Part model, mm, in its own coordinate system. A direction names the side the tool comes from. Give positions to 0.01 mm unless a question says otherwise; leave off trailing zeros. Order: outer loops, then holes, each group sorted by start corner. A loop starts at its lowest first (then second) coordinate and runs counter-clockwise, first axis right, second up. Notation, with made-up numbers: M 16.25,-2 L 38.25,-2 A9 ccw 38.25,12 Z; hole C 37.5,-9 d1. An arc over 180 degrees is marked long. One line per question, with ' | ' between items.
Autodesk Inventor part; units mm, degrees
ref_plane "YZ Plane" through (0, 0, 0) normal (1, 0, 0) x (0, 1, 0)
ref_plane "XZ Plane" through (0, 0, 0) normal (0, 1, 0) x (-1, 0, 0)
ref_plane "XY Plane" through (0, 0, 0) normal (0, 0, 1) x (1, 0, 0)
sketch "Boceto1" plane through (0, 0, 0) normal (0, 0, 1) x (1, 0, 0)
  line L0 (0, 0) -> (-20, 0)
  line L1 (-20, 0) -> (-20, -5)
  line L2 (-20, -5) -> (0, -5)
  line L3 (0, -5) -> (0, 0)
  dimension "d0" = 20
  dimension "d1" = 5
extrude "Extrusión1" add sketch "Boceto1" along normal blind 200
sketch "Boceto2" plane through (-20, 0, 0) normal (0, 1, 0) x (1, 0, 0)
  circle A0 centre (10, -185) radius 2.5
  circle A1 centre (10, -10) radius 2.5
  line L0 (0, 0) -> (0, -200)
  line L1 (0, -15) -> (20, -15) construction
  line L2 (20, 0) -> (0, 0) construction
  dimension "d4" = 5
  dimension "d5" = 5
  dimension "d6" = 10
  dimension "d7" = 10
  dimension "d8" = 15
  dimension "d9" = 10
  dimension "d10" = 170
extrude "Extrusión2" cut sketch "Boceto2" against normal blind 200
sketch "Boceto3" plane through (-20, 0, 0) normal (0, 1, 0) x (1, 0, 0)
  line L0 (20, -200) -> (0, -200)
  line L1 (20, 0) -> (20, -200)
  line L2 (0, -200) -> (20, -200)
  line L3 (20, -200) -> (20, -195)
  line L4 (20, -195) -> (0, -195)
  line L5 (0, -195) -> (0, -200)
  dimension "d13" = 5
extrude "Extrusión3" add sketch "Boceto3" along normal blind 20
sketch "Boceto4" plane through (-20, 0, 0) normal (0, 1, 0) x (1, 0, 0)
  line L0 (20, 0) -> (20, -200)
  line L1 (0, 0) -> (20, 0)
  line L2 (20, 0) -> (20, -5)
  line L3 (20, -5) -> (0, -5)
  line L4 (0, -5) -> (0, 0)
  line L5 (0, 0) -> (0, -200)
  line L6 (0, -15) -> (20, -15)
  line L7 (20, -15) -> (20, -20)
  line L8 (20, -20) -> (0, -20)
  line L9 (0, -20) -> (0, -15)
  dimension "d16" = 5
  dimension "d17" = 5
  dimension "d18" = 10
extrude "Extrusión4" add sketch "Boceto4" along normal blind 10 contours L0 L3 L4 L1 | L0 L8 L5 L6
thread "Rosca1"
thread "Rosca2"
properties part number "Conexión - C15_3DPrint"
1. Drop flat-ended pins along their axis: pin 1 (8 mm diameter, centred on x = -14.5, z = 11.5, fed in from +Y); pin 2 (1 mm diameter, centred on x = -16, z = 76, fed in from +Y). Give the stop position or say it passes through.
Worked out:
pin 1: stops at y = 10 | pin 2: stops at y = 0
2. Slice it at D-D on y = 14.5. Give the cut face in (x, z), then the cut area to 3 significant figures.
Worked out:
outline: M -20,195 L 0,195 L 0,200 L -20,200 Z | area: 100 mm2
3. Slice it at A-A on z = 10. Give the cut face in (x, y), then the cut area to 3 significant figures.
Worked out:
outline: M -20,-5 L -12.5,-5 L -12.5,0 L -20,0 Z; M -7.5,-5 L 0,-5 L 0,0 L -7.5,0 Z | area: 75.0 mm2
4. Slice it at C-C on z = 155.5. Give the cut face in (x, y).
Worked out:
outline: M -20,-5 L 0,-5 L 0,0 L -20,0 Z
5. Probe L1, parallel to Z at x = -10, y = -2.9; L2, parallel to Z at x = -2.5, y = 7; L3, parallel to X at y = -2.25, z = 185. List the from-to ranges inside material, lowest first. Write a range as from..to.
Worked out:
L1: z = 0..7.5, 12.5..182.5, 187.5..200 | L2: z = 0..5, 15..20, 195..200 | L3: x = -20..-12.5, -7.5..0
6. Slice it at B-B on x = -10. Give the cut face in (y, z).
Worked out:
outline: M -5,0 L 10,0 L 10,5 L 0,5 L 0,7.5 L -5,7.5 Z; M -5,12.5 L 0,12.5 L 0,15 L 10,15 L 10,20 L 0,20 L 0,182.5 L -5,182.5 Z; M -5,187.5 L 0,187.5 L 0,195 L 20,195 L 20,200 L -5,200 Z
7. Mould opens along Z. For faces 4 (the flat face through (-7.6, 0, 8.8)), 5 (the flat face through (-10, -5, 99)), 6 (the flat face through (-10, 0, 106)), 7 (the flat face through (-10, 3, 0)) say: released by +Z, released by -Z, zero draft, split by the parting line, or undercut.
Worked out:
face 4: undercut | face 5: zero draft | face 6: undercut | face 7: released by -Z
8. Tool access for faces 1 (the flat face through (-10, 5, 5)), 2 (the flat face through (-10, 10, 17)), 3 (the flat face through (0, -2, 100)): list every direction of +Z, -Z, +X, -X, +Y, -Y with a clear straight run to the whole face (end or side of a thin tool).
Worked out:
face 1: +X, -X, +Y | face 2: -Z, +X, -X, +Y | face 3: +Z, -Z, +X, +Y, -Y
